```python
from build123d import *

# Parameters (mm, degrees)
SKETCH_1_R      = 0.29
EXTRUDE_1_DEPTH = 5
SKETCH_2_W      = 1
SKETCH_2_H      = 1
EXTRUDE_2_DEPTH = 5
SKETCH_3_W      = 1
SKETCH_3_H      = 8
EXTRUDE_3_DEPTH = 0.2
SKETCH_4_R      = 0.95
EXTRUDE_4_DEPTH = 12


with BuildPart() as part:
    # 草图1 → 凸台-拉伸1 (new, symmetric)
    with BuildSketch(Plane(origin=(0, 0, 0), x_dir=(1, 0, 0), z_dir=(0, 1, 0))):
        with Locations(Location((0, 0, 0), (0, 0, 270))):
            Circle(SKETCH_1_R)
    extrude(amount=EXTRUDE_1_DEPTH, both=True)

    # 草图2 → 凸台-拉伸2 (add)
    with BuildSketch(Plane.XY):
        with Locations((0, 4.5)):
            Rectangle(SKETCH_2_W, SKETCH_2_H)
        with Locations((0, -4.5)):
            Rectangle(SKETCH_2_W, SKETCH_2_H)
    extrude(amount=EXTRUDE_2_DEPTH)

    # 草图3 → 凸台-拉伸3 (add)
    with BuildSketch(Plane.XY.offset(5)):
        Rectangle(SKETCH_3_W, SKETCH_3_H)
    extrude(amount=-EXTRUDE_3_DEPTH)

    # 草图4 → 凸台-拉伸4 (add)
    with BuildSketch(Plane.XY.offset(5)):
        with Locations(Location((0, 0, 0), (0, 0, 121.756863859))):
            Circle(SKETCH_4_R)
    extrude(amount=EXTRUDE_4_DEPTH)


solid = part.part
```
Here's how the part is built. I have some questions about the finished solid (model axes, mm). A direction names the side the tool comes from. Coordinates: 2 decimals unless noted, no trailing zeros. Loops run counter-clockwise (first coordinate to the right, second up) from the corner with the lowest first, then second, coordinate; pieces in that order, holes last. Notation, with made-up numbers: (-22, 59) - (-15, 59) arc R12 cw to (-15, 77) - close; hole circle Ø1 at (55.5, -1.5). An arc over 180 degrees is marked (long way). Answer as CSV lines item,"result".
Q1. If we section it at C-C, the plane z = 3: Write out the boundary of the cut face in (x, y), and give its area (3 significant figures).
Response:
outline,"(-0.5, -5) - (0.5, -5) - (0.5, -4) - (-0.5, -4) - close; (-0.5, 4) - (0.5, 4) - (0.5, 5) - (-0.5, 5) - close"
area,"2.00 mm2"
Q2. For pin 1 (0.5 mm diameter, centred on x = -1, y = 0, fed in from -Z); pin 2 (4 mm diameter, centred on y = -2.5, z = 8.5, fed in from -X); pin 3 (0.8 mm diameter, centred on x = 0, y = -4, fed in from +Z), each with a flat end and sliding along its axis, tell me the tip position at first contact or that it passes through.
Response:
pin 1,"z = 5"
pin 2,"x = -0.81"
pin 3,"z = 5"
Q3. If we section it at A-A, the plane y = 0: Write out the boundary of the cut face in (x, z), and give its area (3 significant figures).
Response:
outline,"(-0.95, 5) - (-0.5, 5) - (-0.5, 4.8) - (0.5, 4.8) - (0.5, 5) - (0.95, 5) - (0.95, 17) - (-0.95, 17) - close; circle Ø0.58 at (0, 0)"
area,"23.3 mm2"
Q4. For faces 1 (the face through (-0.177, -0.933, 10.916)), 2 (the face through (0, -5, 2)), which set-ups out of +Z, -Z, +X, -X, +Y, -Y let a thin tool reach every point of the face, with its end or its side?
Response:
face 1,"+Z"
face 2,"+Z, -Z, +X, -X, -Y"
Q5. If we section it at B-B, the plane x = 0: Write out the boundary of the cut face in (y, z), and give its area (3 significant figures).
Response:
outline,"(-5, -0.29) - (5, -0.29) - (5, 5) - (0.95, 5) - (0.95, 17) - (-0.95, 17) - (-0.95, 5) - (-5, 5) - close; hole (-4, 0.29) - (4, 0.29) - (4, 4.8) - (-4, 4.8) - close"
area,"39.6 mm2"
Q6. If we section it at D-D, the plane y = -4.25: Write out the boundary of the cut face in (x, z).
Response:
outline,"(-0.5, 0) - (-0.29, 0) arc R0.29 ccw to (0.29, 0) - (0.5, 0) - (0.5, 5) - (-0.5, 5) - close"
Q7. We'd pull the mould along Y, two halves only. Please class faces 3 (the face through (0, 5, 2)), 4 (the face through (0, -3, 5)), 5 (the face through (0, 0, 4.8)): pulls with the +Y half, pulls with the -Y half, needs draft (parallel to the pull), parting line crosses it, or undercut.
Response:
face 3,"pulls with the +Y half"
face 4,"needs draft"
face 5,"undercut"
Q8. If I drill on L1, parallel to Y at x = -0.35, z = 2; L2, parallel to Z at x = 0.45, y = -1; L3, parallel to Y at x = 0.75, z = 10.5, over which ranges is the centre line in solid material (lowest first)? Write a range as [from, to].
Response:
L1,"[-5, -4], [4, 5]"
L2,"[4.8, 5]"
L3,"[-0.58, 0.58]"
